```python
from build123d import *

# Parameters (mm, degrees)
SKETCH3_R           = 69.85
BOSS_EXTRUDE1_DEPTH = 6.35
SKETCH4_R           = 64.77
CUT_EXTRUDE1_DEPTH  = 3.81
SKETCH5_W           = 44.45
SKETCH5_H           = 25.4
CUT_EXTRUDE2_DEPTH  = 7.35
FILLET1_R           = 10
BOSS_EXTRUDE2_DEPTH = 82.55
BOSS_EXTRUDE3_DEPTH = 127


with BuildPart() as part:
    # Sketch3 → Boss-Extrude1 (new body)
    with BuildSketch(Plane(origin=(0, 0, 0), x_dir=(1, 0, 0), z_dir=(0, 1, 0))):
        Circle(SKETCH3_R)
        with BuildLine():
            Line((-16.448489627, 6.35), (15.301510373, 6.35))
            ThreePointArc((15.301510373, 6.35), (21.651510373, 0), (15.301510373, -6.35))
            Line((15.301510373, -6.35), (-16.448489627, -6.35))
            ThreePointArc((-16.448489627, -6.35), (-22.798489627, 0), (-16.448489627, 6.35))
        make_face(mode=Mode.SUBTRACT)
    extrude(amount=BOSS_EXTRUDE1_DEPTH)

    # Sketch4 → Cut-Extrude1 (cut)
    with BuildSketch(Plane(origin=(0, 6.35, 0), x_dir=(1, 0, 0), z_dir=(0, 1, 0))):
        Circle(SKETCH4_R)
    extrude(amount=-CUT_EXTRUDE1_DEPTH, mode=Mode.SUBTRACT)

    # Sketch5 → Cut-Extrude2 (cut, through all)
    with BuildSketch(Plane(origin=(0, 6.35, 0), x_dir=(1, 0, 0), z_dir=(0, 1, 0))):
        with Locations((0.312165283, -57.905331129)):
            Rectangle(SKETCH5_W, SKETCH5_H)
    extrude(amount=-CUT_EXTRUDE2_DEPTH, mode=Mode.SUBTRACT)

    # Fillet1
    fillet1_edges = [part.edges().sort_by_distance(p)[0] for p in [
        (22.537165283, 1.27, 45.205331129),
        (-21.912834717, 1.27, 45.205331129),
    ]]
    fillet(fillet1_edges, radius=FILLET1_R)

    # Sketch8 → Boss-Extrude2 (add)
    with BuildSketch(Plane.XZ):
        with BuildLine():
            Line((34.258206884, -40.64), (30.448206884, -40.64))
            ThreePointArc((30.448206884, -40.64), (0, -10.191793116), (-30.448206884, -40.64))
            Line((-30.448206884, -40.64), (-34.258206884, -40.64))
            ThreePointArc((-34.258206884, -40.64), (0, -6.381793116), (34.258206884, -40.64))
        make_face()
    extrude(amount=BOSS_EXTRUDE2_DEPTH)

    # Sketch11 → Boss-Extrude3 (add)
    with BuildSketch(Plane(origin=(0, 2.54, 0), x_dir=(1, 0, 0), z_dir=(0, 1, 0))):
        with BuildLine():
            ThreePointArc((-21.912834717, -52.782100893), (-56.087729184, -10.967640358), (-40.18100173, 40.64))
            Line((-40.18100173, 40.64), (-48.791806689, 40.64))
            ThreePointArc((-48.791806689, 40.64), (-61.333240284, -16.446386725), (-21.912834717, -59.599309347))
            Line((-21.912834717, -59.599309347), (-21.912834717, -55.205331129))
            Line((-21.912834717, -55.205331129), (-21.912834717, -52.782100893))
        make_face()
        with BuildLine():
            Line((48.791806689, 40.64), (40.18100173, 40.64))
            ThreePointArc((40.18100173, 40.64), (56.15176968, -10.634907703), (22.537165283, -52.518555588))
            Line((22.537165283, -52.518555588), (22.537165283, -55.205331129))
            Line((22.537165283, -55.205331129), (22.537165283, -59.366035584))
            ThreePointArc((22.537165283, -59.366035584), (61.418705204, -16.124287613), (48.791806689, 40.64))
        make_face()
    extrude(amount=-BOSS_EXTRUDE3_DEPTH)


solid = part.part
```
The listing builds one solid part. Answer for the finished solid, in the listing's coordinates (mm). A direction names the side the tool comes from. Coordinates: 2 decimals unless noted, no trailing zeros. Write each loop counter-clockwise with the first axis right and the second up, starting at its lowest first coordinate (ties: lowest second). Pieces come first, ordered by that corner, then holes. Notation, with made-up numbers: (-38.5, 63.25) -> (-34.5, 63.25) arc R23 cw to (-34.5, 86.25) -> close; hole circle Ø11 at (59.25, 37). An arc over 180 degrees is marked (long way). Write each question's results on one line, items separated by ' | '. Start each with the question number.
1) A cutting plane is placed at D-D (y = -16). Determine the outline of the cut face in (x, z), then the cut area to 3 significant figures.
2) For a pull along Z with two mould halves and no side action, classify faces 1 (the cylindrical face through (56.292, -61.359, 9.865)), 2 (the flat face through (-55, -124.46, 17)), 3 (the cylindrical face through (-19.06, 1.25, 48.21)) as +Z half, -Z half, draft (parallel to the pull), parting line (faces both ways), or undercut.
3) A cutting plane is placed at B-B (y = -115.5). Determine the outline of the cut face in (x, z).
4) Straight lines are drawn through the part: probe 1 along X at (y, z) = (4.2, 0); probe 2 along X at (y, z) = (-77.5, -38.5); probe 3 along X at (y, z) = (-3, -14). For each, find the intervals that lie inside material, in ascending order.
5) Flat-ended cylindrical pins translate along their axes: pin 1 Ø0.8 at (x, y) = (6.5, 1) entering from -Z; pin 2 Ø0.8 at (x, y) = (-2.5, 1) entering from +Z; pin 3 Ø3 at (x, y) = (32, -24.5) entering from -Z; pin 4 Ø10 at (y, z) = (-58.5, -50.5) entering from -X. Find the tip coordinate at first contact, or state that the pin passes through.
6) A cutting plane is placed at A-A (z = 0). Determine the outline of the cut face in (x, y).
7) A tool of negligible diameter and unlimited length cuts with its end or side. For faces 4 (the cylindrical face through (0.7, -40.7, -10.2)), 5 (the cylindrical face through (19.53, 1.252, 48.057)), 6 (the flat face through (32, -41, -40.64)), from which of +Z, -Z, +X, -X, +Y, -Y can it reach the whole face along a straight path? Write none if from no direction.
Values follow:
1) outline: (-48.79, -40.64) -> (-40.18, -40.64) arc R57.15 cw to (-21.91, 52.78) -> (-21.91, 59.6) arc R63.5 ccw to start; (-34.26, -40.64) -> (-30.45, -40.64) arc R30.45 cw to (30.45, -40.64) -> (34.26, -40.64) arc R34.26 ccw to start; (22.54, 52.52) arc R57.15 cw to (40.18, -40.64) -> (48.79, -40.64) arc R63.5 ccw to (22.54, 59.37) -> close | area: 1,870 mm²
2) face 1: undercut | face 2: draft | face 3: +Z half
3) outline: (-48.79, -40.64) -> (-40.18, -40.64) arc R57.15 cw to (-21.91, 52.78) -> (-21.91, 59.6) arc R63.5 ccw to start; (22.54, 52.52) arc R57.15 cw to (40.18, -40.64) -> (48.79, -40.64) arc R63.5 ccw to (22.54, 59.37) -> close
4) probe 1: -69.85 to -64.77, 64.77 to 69.85 | probe 2: -50.5 to -42.24, -34.19 to -30.37, 30.37 to 34.19, 42.24 to 50.5 | probe 3: -61.94 to -55.41, -21.54 to -14.74, 14.74 to 21.54, 55.41 to 61.94
5) pin 1: z = -69.58 | pin 2: z = 45.21 | pin 3: z = -40.64 | pin 4: through
6) outline: (-69.85, 0) -> (-63.5, 0) -> (-63.5, -124.46) -> (-57.15, -124.46) -> (-57.15, 0) -> (-22.8, 0) -> (-22.8, 2.54) -> (-64.77, 2.54) -> (-64.77, 6.35) -> (-69.85, 6.35) -> close; (21.65, 0) -> (57.15, 0) -> (57.15, -124.46) -> (63.5, -124.46) -> (63.5, 0) -> (69.85, 0) -> (69.85, 6.35) -> (64.77, 6.35) -> (64.77, 2.54) -> (21.65, 2.54) -> close
7) face 4: -Z, -Y | face 5: +Z, +Y, -Y | face 6: -Z, +X, -X, -Y
